Autodesk Inventor part; units mm, degrees
ref_plane "YZ Plane" through (0, 0, 0) normal (1, 0, 0) x (0, 1, 0)
ref_plane "XZ Plane" through (0, 0, 0) normal (0, 1, 0) x (-1, 0, 0)
ref_plane "XY Plane" through (0, 0, 0) normal (0, 0, 1) x (1, 0, 0)
sketch "Sketch1" plane through (0, 0, 0) normal (0, 0, 1) x (1, 0, 0)
  line L0 (-50, 48) -> (-50, -15.8)
  line L1 (-50, -15.8) -> (-18.25, -15.8)
  line L2 (-18.25, -15.8) -> (-18.25, -48)
  line L3 (-18.25, -48) -> (18.25, -48)
  line L4 (18.25, -48) -> (18.25, -15.8)
  line L5 (18.25, -15.8) -> (50, -15.8)
  line L6 (50, -15.8) -> (50, 48)
  line L7 (50, 48) -> (-50, 48)
  line L8 (18.25, -48) -> (-18.25, -48)
  line L9 (-18.25, -48) -> (-18.25, -15.8)
  line L10 (-18.25, -15.8) -> (18.25, -15.8)
  line L11 (18.25, -15.8) -> (18.25, -48)
  point P0 (0, 0)
extrude "Extrusion1" add sketch "Sketch1" along normal blind 4.6 contours L10 L4 L3 L2
sketch "Sketch2" plane through (0, 0, 4.6) normal (0, 0, 1) x (1, 0, 0)
  line L0 (-18.25, -15.8) -> (-18.25, -48)
  line L1 (-18.25, -48) -> (18.25, -48)
  line L2 (18.25, -48) -> (18.25, -15.8)
  line L3 (18.25, -15.8) -> (-18.25, -15.8)
  point P0 (0, 0)
extrude "Extrusion2" cut sketch "Sketch2" against normal blind 1
sketch "Sketch3" plane through (0, 0, 0) normal (0, 0, -1) x (-1, 0, 0)
  line L0 (4.9, -29.9) -> (18.1, -29.9)
  line L1 (4.9, -41.9) -> (18.1, -41.9)
  line L2 (-4.9, -41.9) -> (-18.1, -41.9)
  line L3 (-4.9, -29.9) -> (-18.1, -29.9)
  line L4 (11.5, -29.9) -> (11.5, -22.9)
  line L5 (-11.5, -29.9) -> (-11.5, -22.9)
  line L6 (18.25, -15.8) -> (18.25, -48)
  line L7 (-18.25, -15.8) -> (18.25, -15.8)
  line L8 (-18.25, -48) -> (-18.25, -15.8)
  line L9 (18.25, -48) -> (-18.25, -48)
  line L10 (-18.25, -15.8) -> (18.25, -15.8)
  line L11 (0, -15.8) -> (0, -48)
  line L12 (18.25, -48) -> (-18.25, -48)
  line L13 (0, -48) -> (0, -43.5)
  point P0 (0, 0)
  dimension "d4" = 7
  dimension "d5" = 4.5
hole "Hole1" at (-11.5, -22.9, 0) at (11.5, -22.9, 0) direction (0, 0, 1) diameter 3 end through all
sketch "Sketch4" plane through (18.25, -48, 0) normal (1, 0, 0) x (0, 0, -1)
  arc A0 (-8.6, 4.7781) -> (-3.6, -0.73) centre (5, 12.1) ccw
  circle A1 centre (5, 12.1) radius 15.4457
  line L0 (-3.6, 32.2) -> (-3.6, 0)
  line L1 (0, 0) -> (-3.6, 0)
  line L2 (0, 0) -> (0, 32.2)
  line L3 (0, 32.2) -> (-3.6, 32.2)
  line L4 (0, 0) -> (0, -2.514)
  line L5 (-3.6, 0) -> (-3.6, -1.081)
  point P0 (0, 48)
  point P1 (-3.6, -0.73)
extrude "Extrusion3" add sketch "Sketch4" against normal up to surface (36.5 mm away) contours L5 L1 L4 A1
properties part number "podpora silników" material "Lead"
The model under review builds one solid part; all positions refer to its coordinate system, in mm. Round coordinates to 2 decimals unless told otherwise and drop trailing zeros. Write each loop counter-clockwise with the first axis right and the second up, starting at its lowest first coordinate (ties: lowest second). Pieces come first, ordered by that corner, then holes. Notation, with made-up numbers: M -3,16 L 15,16 A11 ccw 15,20 Z; hole C 37,72 d7. An arc over 180 degrees is marked long. Use CSV: the item, a comma, the result in double quotes. Start each with the question number.
(1) Clearance check with a flat-ended pin moving along its axis: P1, Ø2.5, axis at x = -11.5, y = -22.9, coming from the -Z side. State where the tip first meets the part, or that it passes through.
(2) For line 1 along X through (y, z) = (-22.9, 1.45); line 2 along X through (y, z) = (-24, 3.05); line 3 along Y through (x, z) = (-11.5, 1.9), list the stretches that pass through material, from the lowest coordinate up.
(3) The part is to be moulded in two halves that separate along Y. For faces 1 (the face through (0.26, -49.73, 1.88)), 2 (the face through (-11.57, -24.4, 1.83)), 3 (the face through (0, -32, 3.6)), say which applies: +Y half, -Y half, draft (parallel to the pull), parting line (faces both ways), or undercut.
(4) We need section A-A, the plane y = -22.9. State the section outline as (x, z) points, then the cut area to 3 significant figures.
(5) We need section D-D, the plane x = -11.5. State the section outline as (y, z) points.
(6) We need section C-C, the plane z = 2.2. State the section outline as (x, y) points, then the cut area to 3 significant figures.
(7) We need section B-B, the plane x = 12. State the section outline as (y, z) points, then the cut area to 3 significant figures.
Findings:
1,P1,"through"
2,line 1,"-18.25 to -13, -10 to 10, 13 to 18.25"
2,line 2,"-18.25 to -12.52, -10.48 to 10.48, 12.52 to 18.25"
2,line 3,"-49.72 to -24.4, -21.4 to -15.8"
3,face 1,"-Y half"
3,face 2,"undercut"
3,face 3,"draft"
4,outline,"M -18.25,0 L -13,0 L -13,3.6 L -18.25,3.6 Z; M -10,0 L 10,0 L 10,3.6 L -10,3.6 Z; M 13,0 L 18.25,0 L 18.25,3.6 L 13,3.6 Z"
4,area,"110 mm^2"
5,outline,"M -50.51,0 L -24.4,0 L -24.4,3.6 L -48.73,3.6 A15.45 ccw Z; M -21.4,0 L -15.8,0 L -15.8,3.6 L -21.4,3.6 Z"
6,outline,"M -18.25,-49.56 L 18.25,-49.56 L 18.25,-15.8 L -18.25,-15.8 Z; hole C -11.5,-22.9 d3; hole C 11.5,-22.9 d3"
6,area,"1,220 mm^2"
7,outline,"M -50.51,0 L -24.31,0 L -24.31,3.6 L -48.73,3.6 A15.45 ccw Z; M -21.49,0 L -15.8,0 L -15.8,3.6 L -21.49,3.6 Z"
7,area,"112 mm^2"
